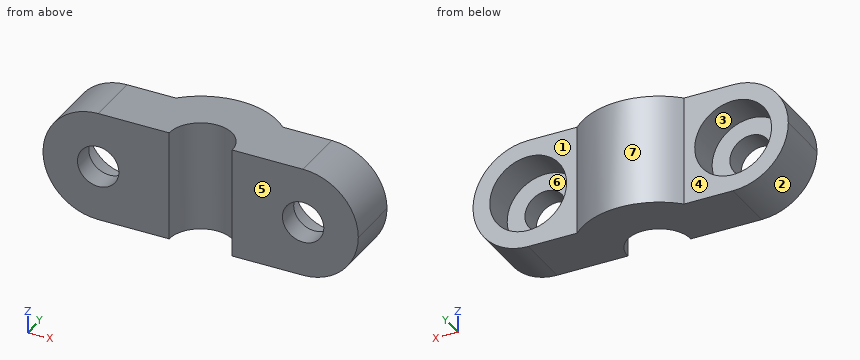
```python
from build123d import *

# Parameters (mm, degrees)
SKETCH1_W           = 40
SKETCH1_H           = 14
BOSS_EXTRUDE1_DEPTH = 7
FILLET1_R           = 7
SKETCH2_R           = 2.625
CUT_EXTRUDE1_DEPTH  = 23.315913604
SKETCH3_R           = 4.875
CUT_EXTRUDE2_DEPTH  = 4.25
BOSS_EXTRUDE2_DEPTH = 14
SKETCH5_R           = 4
CUT_EXTRUDE3_DEPTH  = 27.288067635


with BuildPart() as part:
    # Sketch1 → Boss-Extrude1 (new body)
    with BuildSketch(Plane(origin=(0, 0, 0), x_dir=(1, 0, 0), z_dir=(0, 1, 0))):
        Rectangle(SKETCH1_W, SKETCH1_H)
    extrude(amount=BOSS_EXTRUDE1_DEPTH)

    # Fillet1
    fillet1_edges = [part.edges().sort_by_distance(p)[0] for p in [
        (-20, 3.5, 7),
        (20, 3.5, 7),
        (20, 3.5, -7),
        (-20, 3.5, -7),
    ]]
    fillet(fillet1_edges, radius=FILLET1_R - 0.0001)  # a hair under: the kernel refuses the full size

    # Sketch2 → Cut-Extrude1 (cut, through all)
    with BuildSketch(Plane(origin=(0, 7, 0), x_dir=(1, 0, 0), z_dir=(0, 1, 0))):
        with Locations(Location((-13, 0, 0), (0, 0, 270))):
            Circle(SKETCH2_R)
        with Locations(Location((13, 0, 0), (0, 0, 90))):
            Circle(SKETCH2_R)
    extrude(amount=-CUT_EXTRUDE1_DEPTH, mode=Mode.SUBTRACT)

    # Sketch3 → Cut-Extrude2 (cut)
    with BuildSketch(Plane(origin=(0, 7, 0), x_dir=(1, 0, 0), z_dir=(0, 1, 0))):
        with Locations(Location((-13, 0, 0), (0, 0, 270))):
            Circle(SKETCH3_R)
        with Locations(Location((13, 0, 0), (0, 0, 90))):
            Circle(SKETCH3_R)
    extrude(amount=-CUT_EXTRUDE2_DEPTH, mode=Mode.SUBTRACT)

    # Sketch4 → Boss-Extrude2 (add)
    with BuildSketch(Plane.XY.offset(7)):
        with BuildLine():
            Line((6.78693598, 7), (-6.78693598, 7))
            ThreePointArc((-6.78693598, 7), (0, 9.75), (6.78693598, 7))
        make_face()
    extrude(amount=-BOSS_EXTRUDE2_DEPTH)

    # Sketch5 → Cut-Extrude3 (cut, through all)
    with BuildSketch(Plane.XY.offset(7)):
        Circle(SKETCH5_R)
    extrude(amount=-CUT_EXTRUDE3_DEPTH, mode=Mode.SUBTRACT)


solid = part.part
```
Source: CAD feature listing. Evaluate the final solid. Frame: model axes, mm. Face numbers are marked on the shaded views. A direction names the side the tool comes from. Round coordinates to 2 decimals unless told otherwise and drop trailing zeros. Order: outer loops, then holes, each group sorted by start corner. A loop starts at its lowest first (then second) coordinate and runs counter-clockwise, first axis right, second up. Notation, with made-up numbers: (24.25, -5.5) -> (56.25, -5.5) arc R23 cw to (56.25, 29.5) -> close; hole circle Ø5 at (-29.75, -13). An arc over 180 degrees is marked (long way). One line per item, written item: value. Start each with the question number.
Q1. Draft query along X for the marked faces 5, 6 and 7. Return one class per face: pulls with the +X half, pulls with the -X half, needs draft (parallel to the pull), parting line crosses it, or undercut.
Q2. Access query for the marked faces 1, 2, 3 and 4. Directions: +Z, -Z, +X, -X, +Y, -Y. A direction counts if a zero-diameter tool reaches every point of the face in a straight line with its end or side. Return the directions, or none.
Q3. Section query A-A (y = 1). Give the number of separate pieces and of enclosed holes in the cut face, plus the area to 3 significant figures.
Q4. Section query D-D (x = 0). Return the cut outline in (y, z), plus the area to 3 significant figures.
Q5. Pin query (flat end, axial travel): pin 1 (4 mm diameter, centred on x = -13, z = 0, fed in from -Y); pin 2 (1.5 mm diameter, centred on y = 8.5, z = 5, fed in from -X); pin 3 (4 mm diameter, centred on x = -13.5, z = -3.5, fed in from +Y); pin 4 (4 mm diameter, centred on x = 12, z = -1, fed in from +Y). Return the tip coordinate at first contact, or that it passes through.
Q6. Material intervals for probe 1 along Z at (x, y) = (13, 0.8) (3 decimals); probe 2 along X at (y, z) = (1.9, 0) (3 decimals); probe 3 along X at (y, z) = (6.75, 4), sorted ascending.
Q7. Section query C-C (z = 1.5). Return the cut outline in (x, y).
Findings below:
1. face 5: needs draft
1. face 6: undercut
1. face 7: parting line crosses it
2. face 1: +Z, -Z, +X, +Y
2. face 2: -Z, -X, +Y, -Y
2. face 3: +Y
2. face 4: +Z, -Z, -X, +Y
3. separate pieces: 2
3. enclosed holes: 2
3. area: 366 mm²
4. outline: (4, -7) -> (9.75, -7) -> (9.75, 7) -> (4, 7) -> close
4. area: 80.5 mm²
5. pin 1: through
5. pin 2: x = -5.92
5. pin 3: y = 7
5. pin 4: y = 2.75
6. probe 1: -7 to -2.625, 2.625 to 7
6. probe 2: -20 to -15.625, -10.375 to -3.52, 3.52 to 10.375, 15.625 to 20
6. probe 3: -18.74 to -15.79, -10.21 to 10.21, 15.79 to 18.74
7. outline: (-19.84, 0) -> (-15.15, 0) -> (-15.15, 2.75) -> (-17.64, 2.75) -> (-17.64, 7) -> (-19.84, 7) -> close; (-10.85, 0) -> (-4, 0) arc R4 cw to (4, 0) -> (10.85, 0) -> (10.85, 2.75) -> (8.36, 2.75) -> (8.36, 7) -> (6.79, 7) arc R9.75 ccw to (-6.79, 7) -> (-8.36, 7) -> (-8.36, 2.75) -> (-10.85, 2.75) -> close; (15.15, 0) -> (19.84, 0) -> (19.84, 7) -> (17.64, 7) -> (17.64, 2.75) -> (15.15, 2.75) -> close
